```python
from build123d import *

# Parameters (mm, degrees)
BOSS_EXTRU_1_DEPTH = 10
SKETCH1_R          = 3.55
CUT_EXTRUDE1_DEPTH = 8


with BuildPart() as part:
    # Esquisse1 → Boss.-Extru.1 (new body)
    with BuildSketch(Plane.XY):
        with BuildLine():
            Line((10.599509188, 9.6), (55.599509188, 5.135702408))
            ThreePointArc((55.599509188, 5.135702408), (60.250926744, 0), (55.599509188, -5.135702408))
            Line((55.599509188, -5.135702408), (10.599509188, -9.6))
            ThreePointArc((10.599509188, -9.6), (0, 0), (10.599509188, 9.6))
        make_face()
    extrude(amount=BOSS_EXTRU_1_DEPTH)

    # Sketch1 → Cut-Extrude1 (cut)
    with BuildSketch(Plane(origin=(0, 0, 0), x_dir=(-1, 0, 0), z_dir=(0, 0, -1))):
        with Locations((-10.599509188, 0)):
            Circle(SKETCH1_R)
    extrude(amount=-CUT_EXTRUDE1_DEPTH, mode=Mode.SUBTRACT)


solid = part.part
```
The model under review builds one solid part; all positions refer to its coordinate system, in mm. A direction names the side the tool comes from. Coordinates: 2 decimals unless noted, no trailing zeros. Order: outer loops, then holes, each group sorted by start corner. A loop starts at its lowest first (then second) coordinate and runs counter-clockwise, first axis right, second up. Notation, with made-up numbers: (72.5, -23.5) -> (76.5, -23.5) arc R10 ccw to (76.5, -7.5) -> close; hole circle Ø6 at (53, 13.25). An arc over 180 degrees is marked (long way). Answer in a Markdown table with one row per item. Add a question column.
Item 1: Mouldability with a two-part tool opening along X and no side actions: class faces 3 (the flat face through (32.78, 7.4, 4.93)), 4 (the cylindrical face through (7.213, 1.066, 3.944)), 5 (the flat face through (31, 0, 10)) as +X half, -X half, draft (parallel to the pull), parting line (faces both ways), or undercut.
Item 2: We need section C-C on x = 29.5. Write out the cut boundary in (y, z), plus the area to 3 significant figures.
Item 3: Machinability: for faces 1 (the flat face through (33.415, -7.337, 4.93)), 2 (the flat face through (11, 0, 8)), which of the approach directions +Z, -Z, +X, -X, +Y, -Y give a long, thin tool a straight path to every point of the face, cutting with its end or side? Answer none if there is none.
Item 4: Clearance check with flat-ended pins moving along their axes: pin 1 (4 mm diameter, centred on x = 49.5, z = 4, fed in from -Y); pin 2 (1 mm diameter, centred on y = 3.5, z = 5, fed in from -X); pin 3 (2 mm diameter, centred on y = 3, z = 7.5, fed in from +X); pin 4 (5.5 mm diameter, centred on x = 9.5, y = -1, fed in from -Z). State where each tip first meets the part, or that it passes through.
Item 5: We need section A-A on z = 4.5. Write out the cut boundary in (x, y).
Item 6: To check wall thickness, follow probe 1 along X at (y, z) = (1.5, 1.25); probe 2 along Y at (x, z) = (55.5, 4); probe 3 along X at (y, z) = (2.75, 3.25). State the ranges of each line that lie inside material, in increasing order.
Item 7: We need section B-B on y = 0. Write out the cut boundary in (x, z), plus the area to 3 significant figures.
Item 8: We need section D-D on y = 7.25. Write out the cut boundary in (x, z).
Final values:
| question | item | result |
|---|---|---|
| 1 | face 3 | +X half |
| 1 | face 4 | undercut |
| 1 | face 5 | draft |
| 2 | outline | (-7.72, 0) -> (7.72, 0) -> (7.72, 10) -> (-7.72, 10) -> close |
| 2 | area | 154 mm2 |
| 3 | face 1 | +Z, -Z, +X, -Y |
| 3 | face 2 | -Z |
| 4 | pin 1 | stops at y = -5.94 |
| 4 | pin 2 | stops at x = 0.48 |
| 4 | pin 3 | stops at x = 59.85 |
| 4 | pin 4 | stops at z = 0 |
| 5 | outline | (10.6, -9.6) -> (55.6, -5.14) arc R5.16 ccw to (55.6, 5.14) -> (10.6, 9.6) arc R9.65 ccw (long way) to start; hole circle Ø7.1 at (10.6, 0) |
| 6 | probe 1 | x = 0.12 to 7.38, 13.82 to 60.03 |
| 6 | probe 2 | y = -5.15 to 5.15 |
| 6 | probe 3 | x = 0.4 to 8.35, 12.84 to 59.46 |
| 7 | outline | (0, 0) -> (7.05, 0) -> (7.05, 8) -> (14.15, 8) -> (14.15, 0) -> (60.25, 0) -> (60.25, 10) -> (0, 10) -> close |
| 7 | area | 546 mm2 |
| 8 | outline | (3.28, 0) -> (34.29, 0) -> (34.29, 10) -> (3.28, 10) -> close |
